Read the model definition and answer for the solid it produces. Units are mm, in the model's axes. Coordinates: 2 decimals unless noted, no trailing zeros. Order: outer loops, then holes, each group sorted by start corner. A loop starts at its lowest first (then second) coordinate and runs counter-clockwise, first axis right, second up. Notation, with made-up numbers: (-22.5, -22) -> (6.5, -22) arc R10 cw to (6.5, -15) -> close; hole circle Ø1 at (-38, -39). An arc over 180 degrees is marked (long way). Answer as a JSON object with one key per item and string values. Group by question number.
1) Section C-C on x = 422 is taken. Determine the outline of the cut face in (y, z) (3 decimals), and give its area (3 significant figures).
2) Section B-B on y = 13.5 is taken. Determine the outline of the cut face in (x, z) (3 decimals), and give its area (3 significant figures).
3) Section A-A on z = -52.5 is taken. Determine the outline of the cut face in (x, y) (3 decimals), and give its area (3 significant figures).
4) Consider L1, parallel to Z at x = 601, y = 11 (3 decimals); L2, parallel to Y at x = 260, z = -84 (3 decimals); L3, parallel to Z at x = 606, y = 20.5. Determine where each line is inside the solid, lowest interval first.
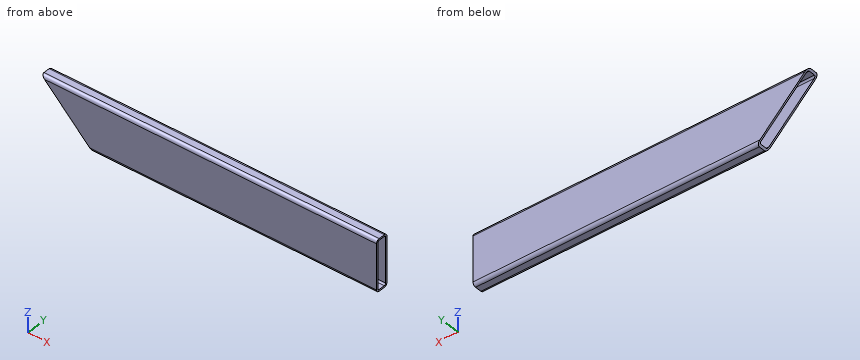
from build123d import *

# Parameters (mm, degrees)
SKETCH1_W           = 101.6
SKETCH1_H           = 25.4
BOSS_EXTRUDE1_DEPTH = 660.4
FILLET1_R           = 6.35
SHELL1_T            = -3.175
CUT_EXTRUDE1_DEPTH  = 25.4


with BuildPart() as part:
    # Sketch1 → Boss-Extrude1 (new body)
    with BuildSketch(Plane(origin=(0, 0, 0), x_dir=(0, 0, -1), z_dir=(1, 0, 0))):
        with Locations((50.8, 12.7)):
            Rectangle(SKETCH1_W, SKETCH1_H)
    extrude(amount=BOSS_EXTRUDE1_DEPTH)

    # Fillet1
    fillet1_edges = [part.edges().sort_by_distance(p)[0] for p in [
        (330.2, 0, 0),
        (330.2, 0, -101.6),
        (330.2, 25.4, -101.6),
        (330.2, 25.4, 0),
    ]]
    fillet(fillet1_edges, radius=FILLET1_R)

    # Shell1
    shell1_openings = [part.faces().sort_by_distance(p)[0] for p in [
        (0, 12.7, -50.8),
        (660.4, 12.7, -50.8),
    ]]
    offset(amount=SHELL1_T, openings=shell1_openings, kind=Kind.INTERSECTION)

    # Sketch2 → Cut-Extrude1 (cut)
    with BuildSketch(Plane(origin=(0, 25.4, 0), x_dir=(1, 0, 0), z_dir=(0, 1, 0))):
        Polygon((0, 0), (101.6, 101.6), (0, 101.6), align=None)
    extrude(amount=-CUT_EXTRUDE1_DEPTH, mode=Mode.SUBTRACT)


solid = part.part
Worked answers:
{
 "1": {"outline": "(0, -95.25) arc R6.35 ccw to (6.35, -101.6) -> (19.05, -101.6) arc R6.35 ccw to (25.4, -95.25) -> (25.4, -6.35) arc R6.35 ccw to (19.05, 0) -> (6.35, 0) arc R6.35 ccw to (0, -6.35) -> close; hole (3.175, -95.25) arc R3.175 ccw to (6.35, -98.425) -> (19.05, -98.425) arc R3.175 ccw to (22.225, -95.25) -> (22.225, -6.35) arc R3.175 ccw to (19.05, -3.175) -> (6.35, -3.175) arc R3.175 ccw to (3.175, -6.35) -> close", "area": "740 mm²"},
 "2": {"outline": "(0, 0) -> (3.175, -3.175) -> (660.4, -3.175) -> (660.4, 0) -> close; (98.425, -98.425) -> (101.6, -101.6) -> (660.4, -101.6) -> (660.4, -98.425) -> close", "area": "3,870 mm²"},
 "3": {"outline": "(52.5, 0) -> (660.4, 0) -> (660.4, 3.175) -> (52.5, 3.175) -> close; (52.5, 22.225) -> (660.4, 22.225) -> (660.4, 25.4) -> (52.5, 25.4) -> close", "area": "3,860 mm²"},
 "4": {"L1": "z = -101.6 to -98.425, -3.175 to 0", "L2": "y = 0 to 3.175, 22.225 to 25.4", "L3": "z = -101.43 to -98.07, -3.53 to -0.17"}
}
